Build history of the part. All positions in model axes, mm. Face numbers are marked on the shaded views. Coordinates: 2 decimals unless noted, no trailing zeros. Order: outer loops, then holes, each group sorted by start corner. A loop starts at its lowest first (then second) coordinate and runs counter-clockwise, first axis right, second up. Notation, with made-up numbers: (-19, 69.25) - (10, 69.25) arc R23 cw to (10, 100.25) - close; hole circle Ø6 at (27, -33.5). An arc over 180 degrees is marked (long way). Return JSON: item names as keys, results as strings.
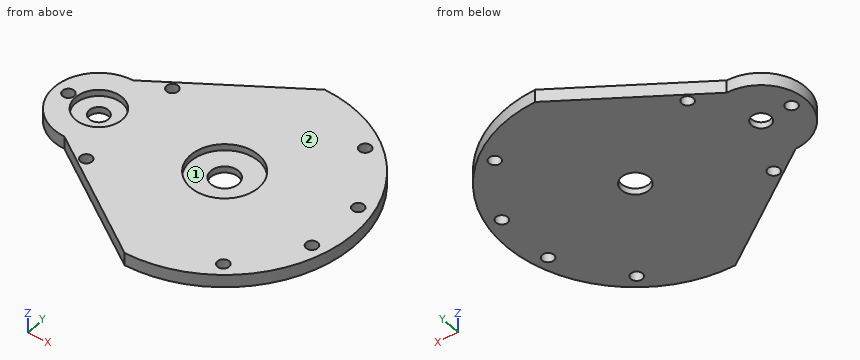
from build123d import *

# Parameters (mm, degrees)
BOSS_EXTRU_1_DEPTH           = 3
ESQUISSE2_R                  = 11
ESQUISSE2_R_2                = 16
ENL_V_MAT_EXTRU_1_DEPTH      = 3
ESQUISSE3_R                  = 4.5
ESQUISSE3_R_2                = 6.5
ENL_V_MAT_EXTRU_2_DEPTH      = 3
ENL_V_MAT_EXTRU_3_DEPTH      = 136.639227364
ENL_V_MAT_EXTRU_3_DEPTH_BACK = 136.639227364
ESQUISSE7_R                  = 2.75


with BuildPart() as part:
    # Esquisse1 → Boss.-Extru.1 (new, symmetric)
    with BuildSketch(Plane.XY):
        with BuildLine():
            Line((0, -21), (60, -61))
            ThreePointArc((60, -61), (121, 0), (60, 61))
            Line((60, 61), (0, 21))
            ThreePointArc((0, 21), (-21, 0), (0, -21))
        make_face()
    extrude(amount=BOSS_EXTRU_1_DEPTH, both=True)

    # Esquisse2 → Enl_v. mat.-Extru.1 (cut)
    with BuildSketch(Plane.XY.offset(3)):
        Circle(ESQUISSE2_R)
        with Locations((60, 0)):
            Circle(ESQUISSE2_R_2)
    extrude(amount=-ENL_V_MAT_EXTRU_1_DEPTH, mode=Mode.SUBTRACT)

    # Esquisse3 → Enl_v. mat.-Extru.2 (cut)
    with BuildSketch(Plane.XY):
        Circle(ESQUISSE3_R)
        with Locations((60, 0)):
            Circle(ESQUISSE3_R_2)
    extrude(amount=-ENL_V_MAT_EXTRU_2_DEPTH, mode=Mode.SUBTRACT)

    # Esquisse7 → Enl_v. mat.-Extru.3 (cut, two sides: drawn at the far end of the back side and taken through both)
    with BuildSketch(Plane(origin=(0, 0, -3), x_dir=(-1, 0, 0), z_dir=(0, 0, -1)).offset(-ENL_V_MAT_EXTRU_3_DEPTH_BACK)):
        with Locations((-93.177497881, 43.237757046)):
            Circle(ESQUISSE7_R)
        with Locations((-112.642957533, 14.105637958)):
            Circle(ESQUISSE7_R)
        with Locations(Location((-93.177497881, -43.237757046, 0), (0, 0, 180))):
            Circle(ESQUISSE7_R)
        with Locations(Location((-112.642957533, -14.105637958, 0), (0, 0, 180))):
            Circle(ESQUISSE7_R)
        with Locations((14.5, 0)):
            Circle(ESQUISSE7_R)
        with Locations((-14.533666301, 26.25)):
            Circle(ESQUISSE7_R)
        with Locations(Location((-14.533666301, -26.25, 0), (0, 0, 180))):
            Circle(ESQUISSE7_R)
    extrude(amount=ENL_V_MAT_EXTRU_3_DEPTH + ENL_V_MAT_EXTRU_3_DEPTH_BACK, mode=Mode.SUBTRACT)


solid = part.part
1. Cut at B-B on y = -26.25. Give the cut face in (x, z) (3 decimals).
Check values:
{"outline": "(7.875, -3) - (11.784, -3) - (11.784, 3) - (7.875, 3) - close; (17.284, -3) - (115.063, -3) - (115.063, 3) - (17.284, 3) - close"}
2. Drop flat-ended pins along their axis: pin 1 (5 mm diameter, centred on x = 93.18, y = 43.24, fed in from -Z); pin 2 (6.5 mm diameter, centred on x = -5, y = -1.5, fed in from +Z); pin 3 (7 mm diameter, centred on x = 14.53, y = -26.25, fed in from -Z); pin 4 (3 mm diameter, centred on y = -19.5, z = -2, fed in from +X). Give the stop position or say it passes through.
Check values:
{"pin 1": "through", "pin 2": "z = 0", "pin 3": "z = -3", "pin 4": "x = 118.28"}
3. Cut at A-A on y = 0. Give the cut face in (x, z).
Check values:
{"outline": "(-21, -3) - (-17.25, -3) - (-17.25, 3) - (-21, 3) - close; (-11.75, -3) - (-4.5, -3) - (-4.5, 0) - (-11, 0) - (-11, 3) - (-11.75, 3) - close; (4.5, -3) - (53.5, -3) - (53.5, 0) - (44, 0) - (44, 3) - (11, 3) - (11, 0) - (4.5, 0) - close; (66.5, -3) - (121, -3) - (121, 3) - (76, 3) - (76, 0) - (66.5, 0) - close"}
4. Cut at D-D on x = 92. Give the cut face in (y, z).
Check values:
{"outline": "(-51.93, -3) - (-45.72, -3) - (-45.72, 3) - (-51.93, 3) - close; (-40.75, -3) - (40.75, -3) - (40.75, 3) - (-40.75, 3) - close; (45.72, -3) - (51.93, -3) - (51.93, 3) - (45.72, 3) - close"}
5. Mould opens along Y. For the marked faces 1 and 2 say: pulls with the +Y half, pulls with the -Y half, needs draft (parallel to the pull), parting line crosses it, or undercut.
Check values:
{"face 1": "undercut", "face 2": "needs draft"}
6. Probe L1, parallel to Y at x = 60, z = -2.1; L2, parallel to Z at x = 53, y = -13.5; L3, parallel to X at y = -12, z = 1.5. List the from-to ranges inside material, lowest first.
Check values:
{"L1": "-61 to -6.5, 6.5 to 61", "L2": "-3 to 0", "L3": "-17.23 to 49.42, 70.58 to 110.87, 114.41 to 119.81"}
7. Cut at C-C on z = 1.35. State how many separate pieces and enclosed holes the cut face has, plus the area to 3 significant figures.
Check values:
{"separate pieces": "1", "enclosed holes": "9", "area": "10,100 mm²"}
